Design review of the part shown in the three views and the two pictorial views. Dimensions are in mm from the part's minimum x, y and z. A direction names the side the tool comes from. Give positions to 0.01 mm unless a question says otherwise; leave off trailing zeros. Loops run counter-clockwise (first coordinate to the right, second up) from the corner with the lowest first, then second, coordinate; pieces in that order, holes last.
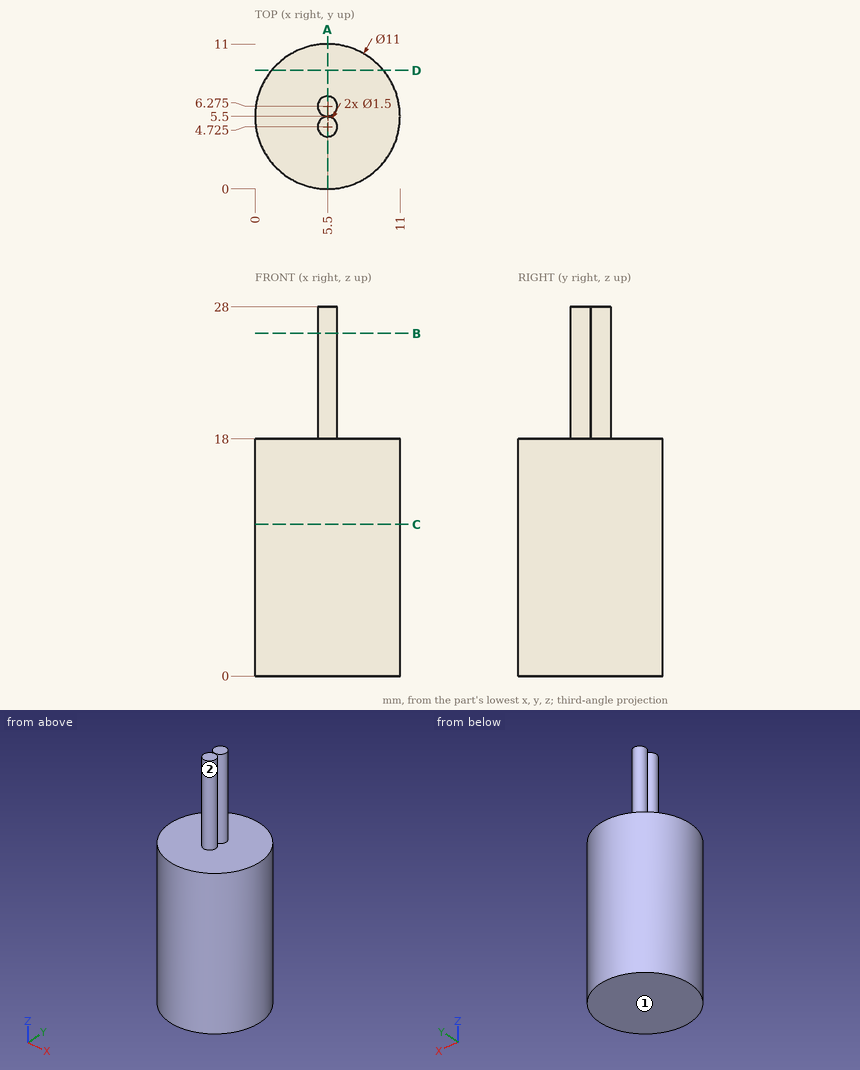
Q1. Take a section at B-B (z = 26). Give the boundary of the cut face in (x, y) (3 decimals).
Results:
outline: circle Ø1.5 at (5.5, 4.725); circle Ø1.5 at (5.5, 6.275)
Q2. Wall thickness on line 1 (Z direction, x = 1.25, y = 8); line 2 (X direction, y = 8, z = 9.5); line 3 (Y direction, x = 6.25, z = 16): over which ranges is each line inside the solid? List them lowest first.
Results:
line 1: z = 0 to 18
line 2: x = 0.6 to 10.4
line 3: y = 0.05 to 10.95
Q3. Take a section at C-C (z = 11.5). Give the boundary of the cut face in (x, y), plus the area to 3 significant figures.
Results:
outline: circle Ø11 at (5.5, 5.5)
area: 95.0 mm2
Q4. Tool access review of the marked faces 1 and 2: name each direction out of +Z, -Z, +X, -X, +Y, -Y from which nothing blocks a thin tool from reaching the whole face with its end or side.
Results:
face 1: -Z, +X, -X, +Y, -Y
face 2: +Z
Q5. Take a section at D-D (y = 9). Give the boundary of the cut face in (x, z), plus the area to 3 significant figures.
Results:
outline: (1.26, 0) - (9.74, 0) - (9.74, 18) - (1.26, 18) - close
area: 153 mm2
Q6. Take a section at A-A (x = 5.5). Give the boundary of the cut face in (y, z) (3 decimals), plus the area to 3 significant figures.
Results:
outline: (0, 0) - (11, 0) - (11, 18) - (7.025, 18) - (7.025, 28) - (5.525, 28) - (5.525, 18) - (5.475, 18) - (5.475, 28) - (3.975, 28) - (3.975, 18) - (0, 18) - close
area: 228 mm2
Q7. Insertion check: pin 1 (1 mm diameter, centred on y = 3, z = 23, fed in from +X); pin 2 (2 mm diameter, centred on x = 7.5, z = 3, fed in from -Y); pin 3 (5 mm diameter, centred on x = 7, z = 24, fed in from -Y) (3 decimals). Each pin has a flat end and moves straight along its axis. Give the tip position at first contact, or say it passes through.
Results:
pin 1: passes through
pin 2: stops at y = 0.09
pin 3: stops at y = 3.975
